Geometry: final body of the model. Coordinates: model frame, mm. A direction names the side the tool comes from. Give positions to 0.01 mm unless a question says otherwise; leave off trailing zeros. Loops run counter-clockwise (first coordinate to the right, second up) from the corner with the lowest first, then second, coordinate; pieces in that order, holes last. Notation, with made-up numbers: (20.5, -20) -> (79.5, -20) arc R19 cw to (79.5, 9) -> close; hole circle Ø1 at (72, 62). An arc over 180 degrees is marked (long way). One line per question, with ' | ' between items. Start each with the question number.
Item 1: Section B-B on x = 38. Return loops of the section in (y, z), then the cut area to 3 significant figures.
Item 2: Pin query (flat end, axial travel): P1, Ø8, axis at y = -24, z = 14, coming from the +X side; P2, Ø5, axis at x = 29, y = -18, coming from the +Z side; P3, Ø6, axis at x = 41, y = -6, coming from the +Z side. Return the tip coordinate at first contact, or that it passes through.
Item 3: Section C-C on y = -20. Return loops of the section in (x, z).
Item 4: Section A-A on z = 8. Return loops of the section in (x, y).
Item 5: Section D-D on x = 23.5. Return loops of the section in (y, z), then the cut area to 3 significant figures.
Item 6: Set-up query: faces 1 (the flat face through (9, -16, 25.4)), 2 (the flat face through (43, -19.05, 10)), 3 (the flat face through (40, -9, 16.51)). Return all of +Z, -Z, +X, -X, +Y, -Y with unobstructed straight access to the full face (end or side cutting, diameter ignored); none if empty.
Item 7: Material intervals for line 1 along Y through (x, z) = (48, 10); line 2 along Z through (x, y) = (39, -3.5); line 3 along X through (y, z) = (-23, 8), sorted ascending. Write a range as [from, to].
from build123d import *

# Parameters (mm, degrees)
F0_W     = 50.8
F0_H     = 25.4
F1_DEPTH = 31.75
F3_DEPTH = 31.75
F5_DEPTH = 19.05


with BuildPart() as f1:
    # F0 (on Front) → F1 (new body)
    with BuildSketch(Plane.XZ):
        with Locations((25.4, 12.7)):
            Rectangle(F0_W, F0_H)
    extrude(amount=F1_DEPTH)

    # F2 (on face) → F3 (cut)
    with BuildSketch(Plane.XZ.offset(31.75)):
        Polygon((50.8, 25.4), (19.05, 25.4), (50.8, 0), align=None)
    extrude(amount=-F3_DEPTH, mode=Mode.SUBTRACT)

    # F4 (on face) → F5 (join)
    with BuildSketch(Plane(origin=(0, 0, 0), x_dir=(-1, 0, 0), z_dir=(0, 1, 0))):
        Polygon((-50.8, 16.51), (-50.8, 0), (-30.1625, 16.51), align=None)
    extrude(amount=-F5_DEPTH)


solid = f1.part
Result sheet:
1) outline: (-31.75, 0) -> (0, 0) -> (0, 16.51) -> (-19.05, 16.51) -> (-19.05, 10.24) -> (-31.75, 10.24) -> close | area: 445 mm²
2) P1: stops at x = 38.3 | P2: stops at z = 19.44 | P3: stops at z = 16.51
3) outline: (0, 0) -> (50.8, 0) -> (19.05, 25.4) -> (0, 25.4) -> close
4) outline: (0, -31.75) -> (40.8, -31.75) -> (40.8, -19.05) -> (50.8, -19.05) -> (50.8, 0) -> (0, 0) -> close
5) outline: (-31.75, 0) -> (0, 0) -> (0, 21.84) -> (-31.75, 21.84) -> close | area: 693 mm²
6) face 1: +Z, +X, -X, +Y, -Y | face 2: +Z, +X, -Y | face 3: +Z, +X, +Y, -Y
7) line 1: y = [-19.05, 0] | line 2: z = [0, 16.51] | line 3: x = [0, 40.8]
